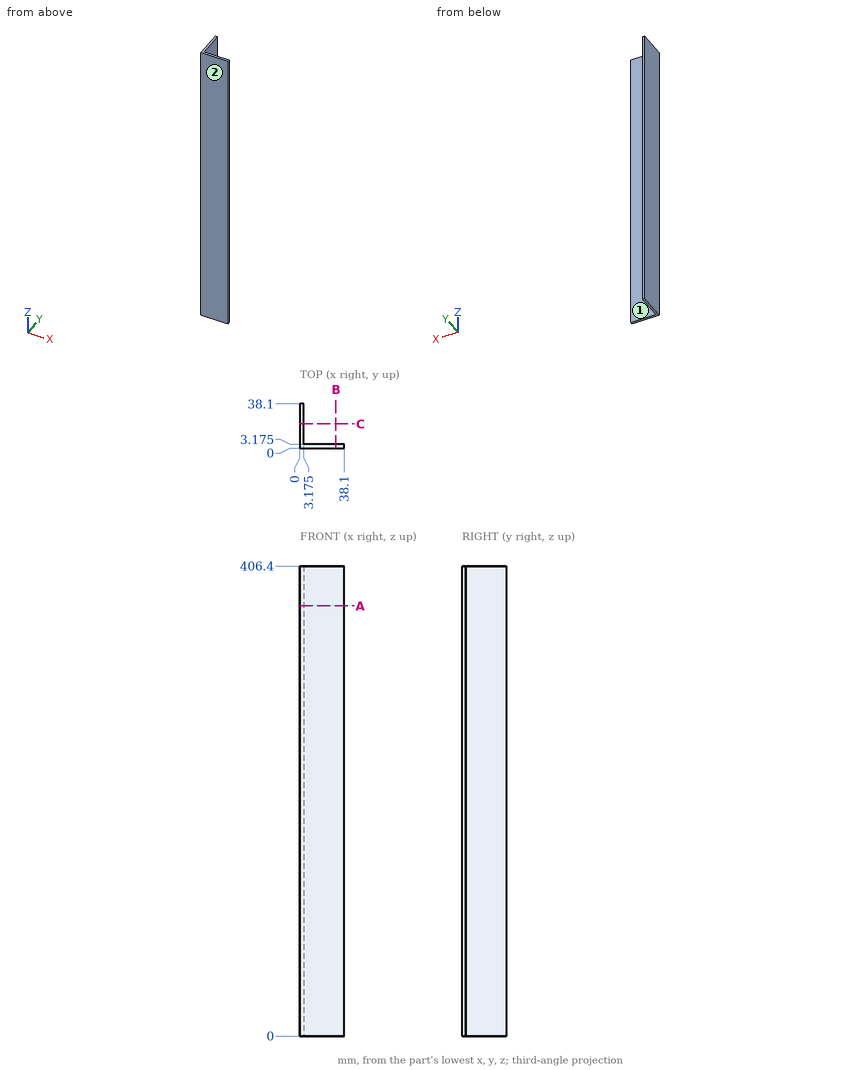
Here's the drawing with two shaded views (mm, measured from the low corner). I have some questions. A direction names the side the tool comes from. Round coordinates to 2 decimals unless told otherwise and drop trailing zeros. Write each loop counter-clockwise with the first axis right and the second up, starting at its lowest first coordinate (ties: lowest second). Pieces come first, ordered by that corner, then holes. Notation, with made-up numbers: M 34.25,38.5 L 89.25,38.5 A16 ccw 89.25,44.5 Z; hole C 50.25,-16.75 d4. An arc over 180 degrees is marked long. Answer in a Markdown table with one row per item. Add a question column.
Q1. Imagine slicing it at B-B (x = 31). Please give me the cut outline in (y, z) (3 decimals), then the cut area to 3 significant figures.
Q2. Imagine slicing it at A-A (z = 372). Please give me the cut outline in (x, y) (3 decimals).
Q3. Will these pins go through, and if not, where does the flat tip stop? pin 1 Ø10.5 at (y, z) = (13.5, 134) entering from +X (3 decimals); pin 2 Ø5 at (x, z) = (15.5, 352) entering from +Y (3 decimals).
Q4. On a 3-axis mill with a long thin cutter (end or side, diameter ignored), from which of +Z, -Z, +X, -X, +Y, -Y can I reach the whole of each face in a straight line? I mean the marked faces 1 and 2. Say none if no direction works.
Q5. If I drill on line 1 (X direction, y = 8.5, z = 245) (3 decimals), over which ranges is the centre line in solid material (lowest first)? Write a range as from..to.
Values:
| question | item | result |
|---|---|---|
| 1 | outline | M 0,0 L 3.175,0 L 3.175,406.4 L 0,406.4 Z |
| 1 | area | 1,290 mm^2 |
| 2 | outline | M 0,0 L 38.1,0 L 38.1,3.175 L 3.175,3.175 L 3.175,38.1 L 0,38.1 Z |
| 3 | pin 1 | x = 3.175 |
| 3 | pin 2 | y = 3.175 |
| 4 | face 1 | +Z, -Z, +X, +Y |
| 4 | face 2 | +Z, -Z, +X, -X, -Y |
| 5 | line 1 | 0..3.175 |
